from build123d import *

# Parameters (mm, degrees)
SKETCH_W     = 32
SKETCH_H     = 20
SKETCH_R     = 1.65
PAD_DEPTH    = 3
SKETCH001_W  = 50.742166
SKETCH001_H  = 6.4
POCKET_DEPTH = 1


with BuildPart() as part:
    # Sketch → Pad (new body)
    with BuildSketch(Plane.XY):
        with Locations((0, -24)):
            Rectangle(SKETCH_W, SKETCH_H)
        with Locations((-11, -17)):
            Circle(SKETCH_R, mode=Mode.SUBTRACT)
        with Locations((11, -17)):
            Circle(SKETCH_R, mode=Mode.SUBTRACT)
        with Locations((-11, -30.4)):
            Circle(SKETCH_R, mode=Mode.SUBTRACT)
        with Locations((11, -30.4)):
            Circle(SKETCH_R, mode=Mode.SUBTRACT)
    extrude(amount=PAD_DEPTH)

    # Sketch001 (on Face10 of Pad) → Pocket (cut)
    with BuildSketch(Plane.XY.offset(3)):
        with Locations((0.273011, -23.7)):
            Rectangle(SKETCH001_W, SKETCH001_H)
    extrude(amount=-POCKET_DEPTH, mode=Mode.SUBTRACT)


solid = part.part
Model file for the job. Use its own axes, mm. A direction names the side the tool comes from. Round coordinates to 2 decimals unless told otherwise and drop trailing zeros. Order: outer loops, then holes, each group sorted by start corner. A loop starts at its lowest first (then second) coordinate and runs counter-clockwise, first axis right, second up.
(1) 3-axis set-ups, long thin cutter, end or side, ignore diameter. For faces 4 (the face through (0, -17, 3)), 5 (the face through (-0.2, -26.9, 2.5)): which of +Z, -Z, +X, -X, +Y, -Y reach the whole face in a straight line?
(2) Band-saw the part on C-C (x = -11). List the corners of the cut face in (y, z), then the cut area to 3 significant figures.
(3) Drill centre lines: line 1 (Y direction, x = 11, z = 1.6); line 2 (Y direction, x = -10.5, z = 2.5); line 3 (X direction, y = -29.75, z = 1.6). Where is each one in solid material? Low to high.
(4) Band-saw the part on B-B (z = 0.4). List the corners of the cut face in (x, y), then the cut area to 3 significant figures.
(5) Band-saw the part on D-D (x = 0.5). List the corners of the cut face in (y, z).
(6) Pull direction X, two halves, no side cores. Call faces 1 (the face through (16, -24, 1)), 2 (the face through (0, -14, 1)), 3 (the face through (11.89, -15.61, 1.48)): released by +X, released by -X, zero draft, split by the parting line, or undercut.
(7) Band-saw the part on A-A (y = -30.4). List the corners of the cut face in (x, z).
Verdict:
1. face 4: +Z, +X, -X, +Y, -Y
1. face 5: +Z, +X, -X
2. outline: (-34, 0) - (-32.05, 0) - (-32.05, 3) - (-34, 3) - close; (-28.75, 0) - (-18.65, 0) - (-18.65, 3) - (-20.5, 3) - (-20.5, 2) - (-26.9, 2) - (-26.9, 3) - (-28.75, 3) - close; (-15.35, 0) - (-14, 0) - (-14, 3) - (-15.35, 3) - close
2. area: 33.8 mm2
3. line 1: y = -34 to -32.05, -28.75 to -18.65, -15.35 to -14
3. line 2: y = -34 to -31.97, -28.83 to -26.9, -20.5 to -18.57, -15.43 to -14
3. line 3: x = -16 to -12.52, -9.48 to 9.48, 12.52 to 16
4. outline: (-16, -34) - (16, -34) - (16, -14) - (-16, -14) - close; hole circle Ø3.3 at (-11, -30.4); hole circle Ø3.3 at (-11, -17); hole circle Ø3.3 at (11, -30.4); hole circle Ø3.3 at (11, -17)
4. area: 606 mm2
5. outline: (-34, 0) - (-14, 0) - (-14, 3) - (-20.5, 3) - (-20.5, 2) - (-26.9, 2) - (-26.9, 3) - (-34, 3) - close
6. face 1: released by +X
6. face 2: zero draft
6. face 3: undercut
7. outline: (-16, 0) - (-12.65, 0) - (-12.65, 3) - (-16, 3) - close; (-9.35, 0) - (9.35, 0) - (9.35, 3) - (-9.35, 3) - close; (12.65, 0) - (16, 0) - (16, 3) - (12.65, 3) - close
